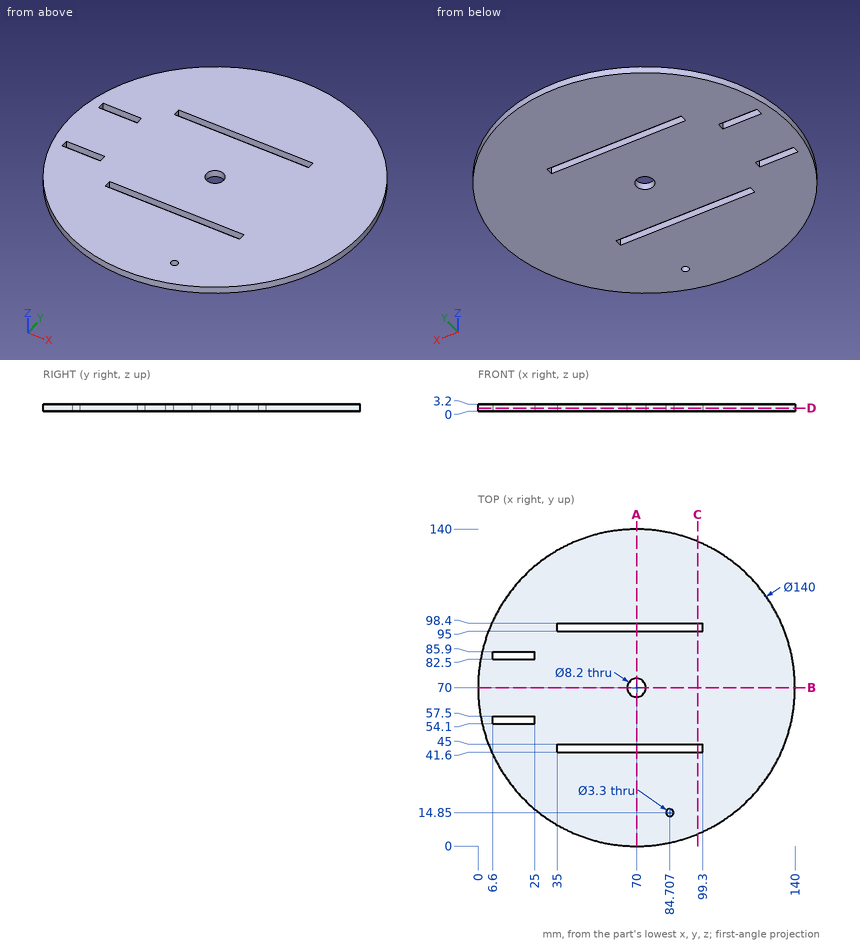
Geometry check sheet. Reference: drawing and pictorial views, mm from the part's lowest x, y, z. Round coordinates to 2 decimals unless told otherwise and drop trailing zeros. Loops run counter-clockwise (first coordinate to the right, second up) from the corner with the lowest first, then second, coordinate; pieces in that order, holes last. Notation, with made-up numbers: (16.25, 4.25) - (65.25, 4.25) arc R27 ccw to (65.25, 33.25) - close; hole circle Ø5 at (-39, 79). An arc over 180 degrees is marked (long way). One line per question, with ' | ' between items. Start each with the question number.
1. Cross-section at C-C on x = 97. Record the cut outline in (y, z).
2. Cross-section at B-B on y = 70. Record the cut outline in (x, z), then the cut area to 3 significant figures.
3. Cross-section at A-A on x = 70. Record the cut outline in (y, z), then the cut area to 3 significant figures.
4. Scan lines: line 1 (Y direction, x = 70, z = 1.3); line 2 (Y direction, x = 82.5, z = 2.75) (1 decimal); line 3 (Y direction, x = 84, z = 1.4) (1 decimal). Record each from-to range of solid material in increasing order. Write a range as [from, to].
5. Cross-section at D-D on z = 1.35. Record the cut outline in (x, y), then the cut area to 3 significant figures.
6. Depth check by flat-ended pin: pin 1 (8 mm diameter, centred on x = 70, y = 48.5, fed in from -Z); pin 2 (1.6 mm diameter, centred on y = 83.5, z = 2, fed in from -X); pin 3 (1.6 mm diameter, centred on y = 97, z = 2.5, fed in from -X); pin 4 (1 mm diameter, centred on y = 44, z = 1.5, fed in from +X). Enter the tip coordinate at first touch or a pass-through.
Taken from the geometry:
1) outline: (5.42, 0) - (41.6, 0) - (41.6, 3.2) - (5.42, 3.2) - close; (45, 0) - (95, 0) - (95, 3.2) - (45, 3.2) - close; (98.4, 0) - (134.58, 0) - (134.58, 3.2) - (98.4, 3.2) - close
2) outline: (0, 0) - (65.9, 0) - (65.9, 3.2) - (0, 3.2) - close; (74.1, 0) - (140, 0) - (140, 3.2) - (74.1, 3.2) - close | area: 422 mm²
3) outline: (0, 0) - (41.6, 0) - (41.6, 3.2) - (0, 3.2) - close; (45, 0) - (65.9, 0) - (65.9, 3.2) - (45, 3.2) - close; (74.1, 0) - (95, 0) - (95, 3.2) - (74.1, 3.2) - close; (98.4, 0) - (140, 0) - (140, 3.2) - (98.4, 3.2) - close | area: 400 mm²
4) line 1: [0, 41.6], [45, 65.9], [74.1, 95], [98.4, 140] | line 2: [1.1, 41.6], [45, 95], [98.4, 138.9] | line 3: [1.4, 13.4], [16.3, 41.6], [45, 95], [98.4, 138.6]
5) outline: circle Ø140 at (70, 70); hole (6.6, 54.1) - (25, 54.1) - (25, 57.5) - (6.6, 57.5) - close; hole (6.6, 82.5) - (25, 82.5) - (25, 85.9) - (6.6, 85.9) - close; hole (35, 41.6) - (99.3, 41.6) - (99.3, 45) - (35, 45) - close; hole (35, 95) - (99.3, 95) - (99.3, 98.4) - (35, 98.4) - close; hole circle Ø8.2 at (70, 70); hole circle Ø3.3 at (84.71, 14.85) | area: 14,800 mm²
6) pin 1: z = 0 | pin 2: x = 1.16 | pin 3: x = 5.09 | pin 4: x = 135.19
